from build123d import *

# Parameters (mm, degrees)
F1_DEPTH = 3.175
F0_W     = 3.175
F0_H     = 12.7
F2_DEPTH = 25.4


with BuildPart() as f1:
    # F0 (on Front) → F1 (new body)
    with BuildSketch(Plane.XZ):
        Polygon((-123.825, 0), (-63.5, 0), (-63.5, 38.1), (-123.825, 38.1), (-123.825, 25.4), (-127, 25.4), (-127, 12.7), (-123.825, 12.7), align=None)
        Polygon((-63.5, 0), (-3.175, 0), (-3.175, 12.7), (0, 12.7), (0, 25.4), (-3.175, 25.4), (-3.175, 38.1), (-63.5, 38.1), align=None)
    extrude(amount=F1_DEPTH)

    # F0 (on Front) → F2 (cut)
    with BuildSketch(Plane.XZ):
        with Locations((-125.4125, 6.35)):
            Rectangle(F0_W, F0_H)
        with Locations((-125.4125, 31.75)):
            Rectangle(F0_W, F0_H)
        with Locations((-1.5875, 31.75)):
            Rectangle(F0_W, F0_H)
        with Locations((-1.5875, 6.35)):
            Rectangle(F0_W, F0_H)
    extrude(amount=-F2_DEPTH, mode=Mode.SUBTRACT)


solid = f1.part
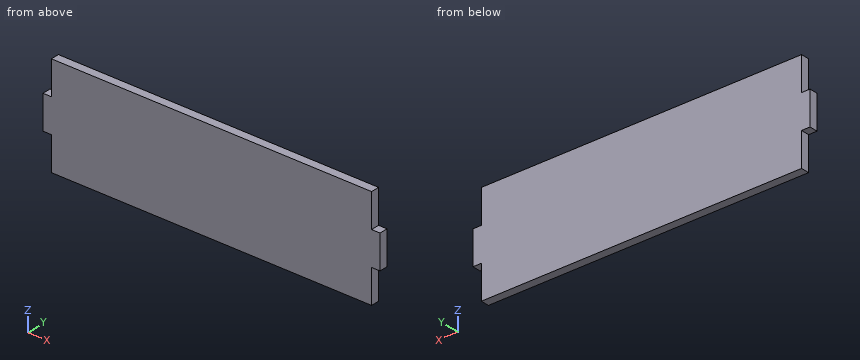
Verification items for the finished model (mm, model axes). Give positions to 0.01 mm unless a question says otherwise; leave off trailing zeros. Loops run counter-clockwise (first coordinate to the right, second up) from the corner with the lowest first, then second, coordinate; pieces in that order, holes last. Notation, with made-up numbers: (46, -34.75) - (84, -34.75) arc R13 cw to (84, -17.75) - close; hole circle Ø6 at (28.25, 12.5). An arc over 180 degrees is marked (long way). Write item = value, one per line. Start each with the question number.
Q1. Depth check by flat-ended pin: P1, Ø1, axis at y = -1, z = 32, coming from the -X side (3 decimals); P2, Ø1.6, axis at y = -2, z = 33.5, coming from the +X side (3 decimals); P3, Ø1.6, axis at x = -125, y = -2, coming from the -Z side. Enter the tip coordinate at first touch or a pass-through.
Q2. Cross-section at B-B, the plane z = 32. Enter the section's corners in (x, y) (3 decimals).
Q3. Cross-section at A-A, the plane y = -1.5. Enter the section's corners in (x, z) (3 decimals).
Q4. Thickness scan on line 1 (X direction, y = -1.6, z = 3.5) (3 decimals). Record the ranges inside material, lowest first.
Answer key:
q1.P1 = -123.825
q1.P2 = -3.175
q1.P3 = 12.7
q2.outline = (-123.825, -3.175) - (-3.175, -3.175) - (-3.175, 0) - (-123.825, 0) - close
q3.outline = (-127, 12.7) - (-123.825, 12.7) - (-123.825, 0) - (-3.175, 0) - (-3.175, 12.7) - (0, 12.7) - (0, 25.4) - (-3.175, 25.4) - (-3.175, 38.1) - (-123.825, 38.1) - (-123.825, 25.4) - (-127, 25.4) - close
q4.line_1 = -123.825 to -3.175
